from build123d import *

# Parameters (mm, degrees)
F1_DEPTH = 3
F2_R     = 2.5
F3_DEPTH = 3


with BuildPart() as f1:
    # F0 (on Top) → F1 (new body)
    with BuildSketch(Plane.XY):
        with BuildLine():
            ThreePointArc((108.2531706913, -187.5000027607), (187.4999986196, -108.2531778639), (216.5063509461, 0))
            ThreePointArc((216.5063509461, 0), (187.4999990763, 108.253177073), (108.2531722731, 187.5000018475))
            ThreePointArc((108.2531722731, 187.5000018475), (1.0905e-06, 216.5063509461), (-108.2531703844, 187.5000029379))
            ThreePointArc((-108.2531703844, 187.5000029379), (-187.4999985558, 108.2531779745), (-216.5063509461, -9.91e-08))
            ThreePointArc((-216.5063509461, -9.91e-08), (-187.4999988892, -108.2531773971), (-108.2531717109, -187.5000021721))
            ThreePointArc((-108.2531717109, -187.5000021721), (-5.886e-07, -216.5063509461), (108.2531706913, -187.5000027607))
        make_face()
        with BuildLine():
            ThreePointArc((-216.5063509461, -9.91e-08), (-187.4999985558, 108.2531779745), (-108.2531703844, 187.5000029379))
            Line((-108.2531703844, 187.5000029379), (-216.5063509461, 125))
            Line((-216.5063509461, 125), (-216.5063509461, -9.91e-08))
        make_face()
        with BuildLine():
            ThreePointArc((-108.2531703844, 187.5000029379), (1.0905e-06, 216.5063509461), (108.2531722731, 187.5000018475))
            Line((108.2531722731, 187.5000018475), (0, 250))
            Line((0, 250), (-108.2531703844, 187.5000029379))
        make_face()
        with BuildLine():
            ThreePointArc((108.2531722731, 187.5000018475), (187.4999990763, 108.253177073), (216.5063509461, 0))
            Line((216.5063509461, 0), (216.5063509461, 125))
            Line((216.5063509461, 125), (108.2531722731, 187.5000018475))
        make_face()
        with BuildLine():
            Line((216.5063509461, -125), (216.5063509461, 0))
            ThreePointArc((216.5063509461, 0), (187.4999986196, -108.2531778639), (108.2531706913, -187.5000027607))
            Line((108.2531706913, -187.5000027607), (216.5063509461, -125))
        make_face()
        with BuildLine():
            Line((0, -250), (108.2531706913, -187.5000027607))
            ThreePointArc((108.2531706913, -187.5000027607), (-5.886e-07, -216.5063509461), (-108.2531717109, -187.5000021721))
            Line((-108.2531717109, -187.5000021721), (0, -250))
        make_face()
        with BuildLine():
            Line((-216.5063509461, -125), (-108.2531717109, -187.5000021721))
            ThreePointArc((-108.2531717109, -187.5000021721), (-187.4999988892, -108.2531773971), (-216.5063509461, -9.91e-08))
            Line((-216.5063509461, -9.91e-08), (-216.5063509461, -125))
        make_face()
    extrude(amount=-F1_DEPTH)

    # F2 (on face) → F3 (cut, through all)
    with BuildSketch(Plane.XY):
        with Locations((-65, 0)):
            Circle(F2_R)
        with Locations((32.5, -56.291651246)):
            Circle(F2_R)
        with Locations((6.7943501124, -64.6439231989)):
            Circle(F2_R)
        with Locations((-20.0861046344, -61.8186735592)):
            Circle(F2_R)
        with Locations((-43.4934894133, -48.304413656)):
            Circle(F2_R)
        with Locations((-59.3804547468, -26.4378817999)):
            Circle(F2_R)
        with Locations((-59.3804547468, 26.4378817999)):
            Circle(F2_R)
        with Locations((-43.4934894133, 48.304413656)):
            Circle(F2_R)
        with Locations((-20.0861046344, 61.8186735592)):
            Circle(F2_R)
        with Locations((6.7943501124, 64.6439231989)):
            Circle(F2_R)
        with Locations((32.5, 56.291651246)):
            Circle(F2_R)
        with Locations((52.5861046344, 38.206041399)):
            Circle(F2_R)
        with Locations((63.5795940477, 13.5142599032)):
            Circle(F2_R)
        with Locations((63.5795940477, -13.5142599032)):
            Circle(F2_R)
        with Locations((52.5861046344, -38.206041399)):
            Circle(F2_R)
    extrude(amount=-F3_DEPTH, mode=Mode.SUBTRACT)


solid = f1.part
Work out the finished part from the listing and answer in its coordinate system (mm). Round coordinates to 2 decimals unless told otherwise and drop trailing zeros. Loops run counter-clockwise (first coordinate to the right, second up) from the corner with the lowest first, then second, coordinate; pieces in that order, holes last. Notation, with made-up numbers: (43, -16.75) - (93, -16.75) arc R22 ccw to (93, 10.25) - close; hole circle Ø2 at (85.5, 23). An arc over 180 degrees is marked (long way). Use one line per item in the form item = value. Start each with the question number.
(1) Find section C-C on y = 167.5. Determine the outline of the cut face in (x, z).
(2) Find section A-A on z = -1.45. Give the number of separate pieces and of enclosed holes in the cut face, and give its area (3 significant figures).
(3) Flat-ended cylindrical pins translate along their axes: P1, Ø1, axis at x = -78, z = -2, coming from the -Y side; P2, Ø1.5, axis at x = -43.5, z = -1.5, coming from the +Y side. Find the tip coordinate at first contact, or state that the pin passes through.
(4) Consider line 1 (X direction, y = 62.5, z = -1.35); line 2 (X direction, y = -56.5, z = -2.45); line 3 (Y direction, x = 24, z = -2.1). Determine where each line is inside the solid, lowest interval first.
(5) Find section B-B on x = -123. Determine the outline of the cut face in (y, z), and give its area (3 significant figures).
Answer list:
q1.outline = (-142.89, -3) - (142.89, -3) - (142.89, 0) - (-142.89, 0) - close
q2.separate_pieces = 1
q2.enclosed_holes = 15
q2.area = 162,000 mm^2
q3.P1 = -205.26
q3.P2 = 225.32
q4.line_1 = -216.51 to -22.49, -17.68 to 5.51, 8.08 to 216.51
q4.line_2 = -216.51 to 30.01, 34.99 to 216.51
q4.line_3 = -236.14 to 236.14
q5.outline = (-178.99, -3) - (178.99, -3) - (178.99, 0) - (-178.99, 0) - close
q5.area = 1,070 mm^2
